Print and shaded views of the part. All mm, measured from the part's lowest x, y and z. Coordinates: 2 decimals unless noted, no trailing zeros. Order: outer loops, then holes, each group sorted by start corner. A loop starts at its lowest first (then second) coordinate and runs counter-clockwise, first axis right, second up. Notation, with made-up numbers: (72.5, -5.75) -> (106.5, -5.75) arc R13 cw to (106.5, 11.25) -> close; hole circle Ø6 at (54.25, -21). An arc over 180 degrees is marked (long way). Write item = value, one per line. Start each with the question number.
Q1. Cut at C-C, the plane z = 8. List the corners of the cut face in (x, y), plus the area to 3 significant figures.
Q2. Cut at B-B, the plane y = 1.25. List the corners of the cut face in (x, z).
Q3. Cut at A-A, the plane x = 25.5. List the corners of the cut face in (y, z).
Q4. Wall check: line 1 (Z direction, x = 24, y = 1.45); line 2 (Z direction, x = 16, y = 1.2); line 3 (X direction, y = 1.05, z = 7.25). Give the ranges that are in metal, low to high. Write a range as from..to.
Q5. Cut at D-D, the plane z = 13.75. List the corners of the cut face in (x, y).
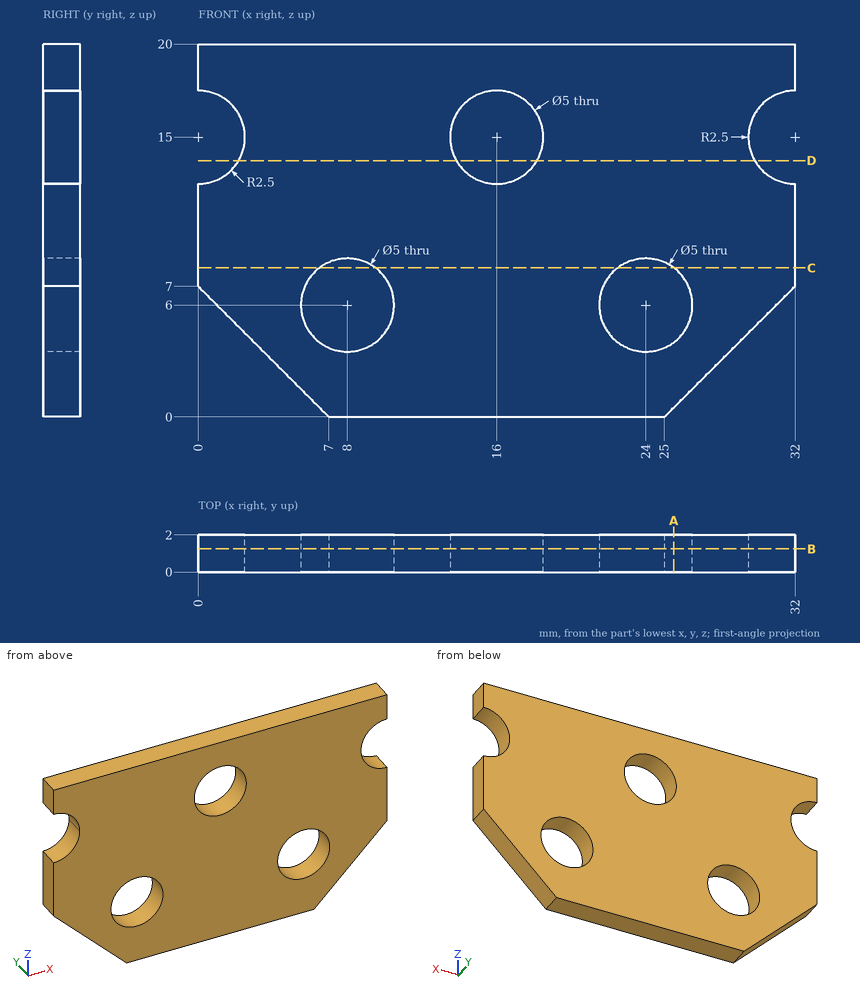
Here are the results:
q1.outline = (0, 0) -> (6.5, 0) -> (6.5, 2) -> (0, 2) -> close; (9.5, 0) -> (22.5, 0) -> (22.5, 2) -> (9.5, 2) -> close; (25.5, 0) -> (32, 0) -> (32, 2) -> (25.5, 2) -> close
q1.area = 52.0 mm²
q2.outline = (0, 7) -> (7, 0) -> (25, 0) -> (32, 7) -> (32, 12.5) arc R2.5 cw to (32, 17.5) -> (32, 20) -> (0, 20) -> (0, 17.5) arc R2.5 cw to (0, 12.5) -> close; hole circle Ø5 at (8, 6); hole circle Ø5 at (16, 15); hole circle Ø5 at (24, 6)
q3.outline = (0, 0.5) -> (2, 0.5) -> (2, 4) -> (0, 4) -> close; (0, 8) -> (2, 8) -> (2, 20) -> (0, 20) -> close
q4.line_1 = 0..3.5, 8.5..20
q4.line_2 = 0..12.5, 17.5..20
q4.line_3 = 0..5.83, 10.17..21.83, 26.17..32
q5.outline = (2.17, 0) -> (13.83, 0) -> (13.83, 2) -> (2.17, 2) -> close; (18.17, 0) -> (29.83, 0) -> (29.83, 2) -> (18.17, 2) -> close
